Check sheet for the modelled part. Datum: model origin and axes. Units: mm. A direction names the side the tool comes from. Round coordinates to 2 decimals unless told otherwise and drop trailing zeros. Loops run counter-clockwise (first coordinate to the right, second up) from the corner with the lowest first, then second, coordinate; pieces in that order, holes last. Notation, with made-up numbers: (-10.75, 29) - (3.25, 29) arc R21 ccw to (3.25, 65) - close; hole circle Ø8 at (89.25, 86). An arc over 180 degrees is marked (long way). Put each result on its own line as item: value.
```python
from build123d import *

# Parameters (mm, degrees)
SKETCH1_R                    = 40
SKETCH1_R_2                  = 27.5
BOSS_EXTRUDE1_DEPTH          = 40
SKETCH3_R                    = 60
BOSS_EXTRUDE2_DEPTH          = 20
SKETCH4_R                    = 30
SKETCH4_R_2                  = 5
CUT_EXTRUDE2_DEPTH           = 90
CHAMFER2_SIZE                = 9
CHAMFER2_SIZE2               = 10.725782333
CUT_EXTRUDE_THIN2_DEPTH      = 2
CUT_EXTRUDE_THIN2_DEPTH_BACK = 1
SKETCH6_R                    = 55.520808166
SKETCH6_R_2                  = 45.520808166


with BuildPart() as part:
    # Sketch1 → Boss-Extrude1 (new body)
    with BuildSketch(Plane.XY):
        Circle(SKETCH1_R)
        Circle(SKETCH1_R_2, mode=Mode.SUBTRACT)
    extrude(amount=BOSS_EXTRUDE1_DEPTH)

    # Sketch3 → Boss-Extrude2 (add)
    with BuildSketch(Plane.XY.offset(40)):
        Circle(SKETCH3_R)
    extrude(amount=BOSS_EXTRUDE2_DEPTH)

    # Sketch4 → Cut-Extrude2 (cut)
    with BuildSketch(Plane.XY.offset(60)):
        Circle(SKETCH4_R)
        with Locations((0, 45.541587837)):
            Circle(SKETCH4_R_2)
        with Locations((39.404155872, 22.791587837)):
            Circle(SKETCH4_R_2)
        with Locations((39.404155872, -22.708412163)):
            Circle(SKETCH4_R_2)
        with Locations((0, -45.458412163)):
            Circle(SKETCH4_R_2)
        with Locations((-39.404155872, -22.708412163)):
            Circle(SKETCH4_R_2)
        with Locations((-39.404155872, 22.791587837)):
            Circle(SKETCH4_R_2)
    extrude(amount=-CUT_EXTRUDE2_DEPTH, mode=Mode.SUBTRACT)

    # Chamfer2
    chamfer2_edges = [part.edges().sort_by_distance(p)[0] for p in [
        (-60, 0, 40),
    ]]
    chamfer2_side = [part.faces().sort_by_distance(p)[0] for p in [
        (-58.302943725, 0, 40),
    ]]
    chamfer(chamfer2_edges, length=CHAMFER2_SIZE, length2=CHAMFER2_SIZE2, reference=chamfer2_side[0])

    # Sketch6 → Cut-Extrude-Thin2 (cut, two sides: drawn at the far end of the back side and taken through both)
    with BuildSketch(Plane.XY.offset(60).offset(-CUT_EXTRUDE_THIN2_DEPTH_BACK)):
        Circle(SKETCH6_R)
        Circle(SKETCH6_R_2, mode=Mode.SUBTRACT)
    extrude(amount=CUT_EXTRUDE_THIN2_DEPTH + CUT_EXTRUDE_THIN2_DEPTH_BACK, mode=Mode.SUBTRACT)


solid = part.part
```
Item 1: Go/stop test with flat-tipped pins: pin 1 (2 mm diameter, centred on x = 35.5, y = -19.5, fed in from -Z); pin 2 (8 mm diameter, centred on x = -39.4, y = -22.71, fed in from +Z); pin 3 (3 mm diameter, centred on y = 22, z = 50, fed in from +X); pin 4 (10 mm diameter, centred on x = -43.5, z = 52, fed in from -Y). Record where each tip stops, or that it passes through.
Filled sheet:
pin 1: z = 0
pin 2: through
pin 3: x = 56.32
pin 4: y = -46.02
Item 2: Section check D-D on y = 20.5. Count the separate pieces of the cut face and the enclosed holes in it, then the cut area to 3 significant figures.
Filled sheet:
separate pieces: 4
enclosed holes: 0
area: 1,900 mm²
Item 3: Section check B-B on y = 0. Enter the section's corners in (x, z), then the cut area to 3 significant figures.
Filled sheet:
outline: (-60, 50.73) - (-51, 40) - (-40, 40) - (-40, 0) - (-30, 0) - (-30, 60) - (-45.52, 60) - (-45.52, 59) - (-55.52, 59) - (-55.52, 60) - (-60, 60) - close; (30, 0) - (40, 0) - (40, 40) - (51, 40) - (60, 50.73) - (60, 60) - (55.52, 60) - (55.52, 59) - (45.52, 59) - (45.52, 60) - (30, 60) - close
area: 1,880 mm²
Item 4: Thickness scan on line 1 (Y direction, x = -40.5, z = 46) (3 decimals); line 2 (Z direction, x = -40, y = -29); line 3 (Z direction, x = -40.5, y = 9.5). Record the ranges inside material, lowest first. Write a range as from..to.
Filled sheet:
line 1: -38.725..-27.587, -17.83..17.913, 27.67..38.725
line 2: 40..59
line 3: 40..60
Item 5: Section check A-A on x = 0. Enter the section's corners in (y, z), then the cut area to 3 significant figures.
Filled sheet:
outline: (-60, 50.73) - (-51, 40) - (-50.46, 40) - (-50.46, 59) - (-55.52, 59) - (-55.52, 60) - (-60, 60) - close; (-40.46, 40) - (-40, 40) - (-40, 0) - (-30, 0) - (-30, 60) - (-40.46, 60) - close; (30, 0) - (40, 0) - (40, 40) - (40.54, 40) - (40.54, 60) - (30, 60) - close; (50.54, 40) - (51, 40) - (60, 50.73) - (60, 60) - (55.52, 60) - (55.52, 59) - (50.54, 59) - close
area: 1,490 mm²
Item 6: Release check for a two-part mould opening along X. For faces 4 (the flat face through (15, -38, 40)), 5 (the conical face through (-11.178, -50.337, 40.671)), 6 (the cylindrical face through (22.548, -39.544, 59.493)) record: +X half, -X half, draft (parallel to the pull), parting line (faces both ways), or undercut.
Filled sheet:
face 4: draft
face 5: parting line
face 6: undercut
Item 7: Tool access check on faces 1 (the cylindrical face through (-8.67, -39.05, 19.72)), 2 (the cylindrical face through (45.52, -0.23, 59.49)), 3 (the cylindrical face through (35.72, -19.33, 50.14)). Record the directions out of +Z, -Z, +X, -X, +Y, -Y that give a thin tool (end or side, any length) a straight path to the whole face; none if there is none.
Filled sheet:
face 1: -Z
face 2: +Z
face 3: +Z, -Z
Item 8: Section check C-C on z = 31.5. Enter the section's corners in (x, y).
Filled sheet:
outline: circle Ø80 at (0, 0); hole circle Ø60 at (0, 0)
